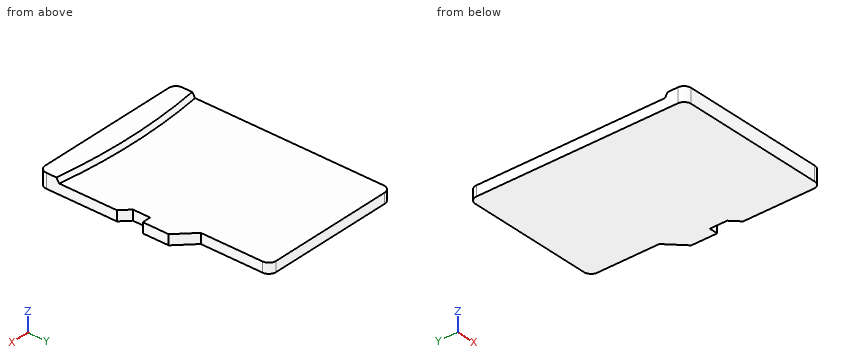
```python
from build123d import *

# Parameters (mm, degrees)
BOX072_W         = 11
BOX072_H         = 15
BOX072_DEPTH     = 0.3
EXTRUDE017_DEPTH = 1


with BuildPart() as cone:
    # Cone → Cone (revolve)
    with BuildSketch(Plane(origin=(0, -36.4, 0.7), x_dir=(1, 0, 0), z_dir=(0, -1, 0))):
        Polygon((0, 0), (38.2, 0), (38, 0.3), (0, 0.3), align=None)
    revolve(axis=Axis((0, -36.4, 0.7), (0, 0, 1)))


with BuildPart() as cut018:
    # Box072 → Box072 (new body)
    with BuildSketch(Plane(origin=(-5.5, 0, 0.7), x_dir=(1, 0, 0), z_dir=(0, 0, 1))):
        with Locations((5.5, 7.5)):
            Rectangle(BOX072_W, BOX072_H)
    extrude(amount=BOX072_DEPTH)

    # Cut018: cut Cone
    add(cone.part, mode=Mode.SUBTRACT)


with BuildPart() as body:
    # Sketch018 → Extrude017 (new body)
    with BuildSketch(Plane.XY):
        with BuildLine():
            Line((-5.5, 0.5), (-5.5, 14.5))
            ThreePointArc((-5, 15), (-5.353553, 14.853553), (-5.5, 14.5))
            Line((-5, 15), (3.8, 15))
            ThreePointArc((4.3, 14.5), (4.153553, 14.853553), (3.8, 15))
            Line((4.3, 14.5), (4.3, 10.2))
            Line((4.3, 10.2), (5.5, 9))
            Line((5.5, 9), (5.5, 7.2))
            Line((5.5, 7.2), (4.9, 7.2))
            Line((4.9, 7.2), (4.9, 6))
            Line((4.9, 6), (5.5, 5.4))
            Line((5.5, 5.4), (5.5, 0.5))
            ThreePointArc((5, 0), (5.353553, 0.146447), (5.5, 0.5))
            Line((5, 0), (-5, 0))
            ThreePointArc((-5.5, 0.5), (-5.353553, 0.146447), (-5, 0))
        make_face()
    extrude(amount=EXTRUDE017_DEPTH)

    # Cut019: cut Cut018
    add(cut018.part, mode=Mode.SUBTRACT)


solid = body.part
```
The model under review builds one solid part; all positions refer to its coordinate system, in mm. Give positions to 0.01 mm unless a question says otherwise; leave off trailing zeros. Loops run counter-clockwise (first coordinate to the right, second up) from the corner with the lowest first, then second, coordinate; pieces in that order, holes last. Notation, with made-up numbers: (50.5, 39) -> (98.5, 39) arc R14 ccw to (98.5, 60) -> close; hole circle Ø11 at (-6, -1.75). An arc over 180 degrees is marked (long way). Use CSV: the item, a comma, the result in double quotes.
1. Consider section C-C, the plane y = 6.75. Write out the cut boundary in (x, z).
Result:
outline,"(-5.5, 0) -> (4.9, 0) -> (4.9, 0.7) -> (-5.5, 0.7) -> close"
2. Consider section B-B, the plane y = 3.25. Write out the cut boundary in (x, z).
Result:
outline,"(-5.5, 0) -> (5.5, 0) -> (5.5, 0.7) -> (-5.5, 0.7) -> close"
3. To check wall thickness, follow probe 1 along Z at (x, y) = (3, 4.75); probe 2 along X at (y, z) = (10.5, 0.25); probe 3 along Y at (x, z) = (-4.5, 0.9). State the ranges of each line that lie inside material, in increasing order. Write a range as from..to.
Result:
probe 1,"z = 0..0.7"
probe 2,"x = -5.5..4.3"
probe 3,"y = 0..1.4"
4. For P1, Ø1.5, axis at x = -3, y = 2.5, coming from the +Z side; P2, Ø0.6, axis at y = 13, z = 0.5, coming from the +X side, all flat-tipped, find the tip position at first contact; note any pin that passes through.
Result:
P1,"stops at z = 0.7"
P2,"stops at x = 4.3"
5. Consider section A-A, the plane z = 0.15. Write out the cut boundary in (x, y), then the cut area to 3 significant figures.
Result:
outline,"(-5.5, 0.5) arc R0.5 ccw to (-5, 0) -> (5, 0) arc R0.5 ccw to (5.5, 0.5) -> (5.5, 5.4) -> (4.9, 6) -> (4.9, 7.2) -> (5.5, 7.2) -> (5.5, 9) -> (4.3, 10.2) -> (4.3, 14.5) arc R0.5 ccw to (3.8, 15) -> (-5, 15) arc R0.5 ccw to (-5.5, 14.5) -> close"
area,"157 mm²"
